```python
from build123d import *

# Parameters (mm, degrees)
SKETCH1_R           = 2.54
BOSS_EXTRUDE1_DEPTH = 0.8128
SKETCH2_R           = 2.54
CUT_EXTRUDE1_DEPTH  = 118.606454516
SKETCH3_R           = 2.54
CUT_EXTRUDE2_DEPTH  = 118.606454516


with BuildPart() as part:
    # Sketch1 → Boss-Extrude1 (new body)
    with BuildSketch(Plane(origin=(0, 0, 0), x_dir=(1, 0, 0), z_dir=(0, 1, 0))):
        Polygon((0, 88.9), (-76.989658396, 44.45), (-76.989658396, -44.45), (0, -88.9), (76.989658396, -44.45), (76.989658396, 44.45), align=None)
        with Locations(Location((13.322783942, -73.875738686, 0), (0, 0, 270))):
            Circle(SKETCH1_R, mode=Mode.SUBTRACT)
        with Locations(Location((24.32130657, -67.525738686, 0), (0, 0, 270))):
            Circle(SKETCH1_R, mode=Mode.SUBTRACT)
        with Locations(Location((-70.639658396, 12.7, 0), (0, 0, 270))):
            Circle(SKETCH1_R, mode=Mode.SUBTRACT)
        with Locations(Location((-70.639658396, 25.4, 0), (0, 0, 270))):
            Circle(SKETCH1_R, mode=Mode.SUBTRACT)
        with Locations(Location((46.318351826, 54.825738686, 0), (0, 0, 270))):
            Circle(SKETCH1_R, mode=Mode.SUBTRACT)
        with Locations(Location((57.316874454, 48.475738686, 0), (0, 0, 270))):
            Circle(SKETCH1_R, mode=Mode.SUBTRACT)
    extrude(amount=BOSS_EXTRUDE1_DEPTH)

    # Sketch2 → Cut-Extrude1 (cut, through all)
    with BuildSketch(Plane(origin=(0, 0.8128, 0), x_dir=(1, 0, 0), z_dir=(0, 1, 0))):
        with Locations(Location((28.620590949, 59.732317666, 0), (0, 0, 270))):
            Circle(SKETCH2_R)
        with Locations(Location((48.416295038, -22.82051708, 0), (0, 0, 270))):
            Circle(SKETCH2_R)
        with Locations(Location((-52.77011314, 35.59948292, 0), (0, 0, 270))):
            Circle(SKETCH2_R)
        with Locations(Location((-32.974409051, -46.953351826, 0), (0, 0, 270))):
            Circle(SKETCH2_R)
    extrude(amount=-CUT_EXTRUDE1_DEPTH, mode=Mode.SUBTRACT)

    # Sketch3 → Cut-Extrude2 (cut, through all)
    with BuildSketch(Plane(origin=(0, 0.8128, 0), x_dir=(1, 0, 0), z_dir=(0, 1, 0))):
        with Locations(Location((-7.823522628, -77.050738686, 0), (0, 0, 270))):
            Circle(SKETCH3_R)
        with Locations(Location((-62.816135768, -45.300738686, 0), (0, 0, 270))):
            Circle(SKETCH3_R)
        with Locations(Location((-56.466135768, -34.302216058, 0), (0, 0, 270))):
            Circle(SKETCH3_R)
        with Locations(Location((-1.473522628, -66.052216058, 0), (0, 0, 270))):
            Circle(SKETCH3_R)
    extrude(amount=-CUT_EXTRUDE2_DEPTH, mode=Mode.SUBTRACT)


solid = part.part
```
CAD build for the part. Positions are in the model's coordinates, mm. Round coordinates to 2 decimals unless told otherwise and drop trailing zeros. Write each loop counter-clockwise with the first axis right and the second up, starting at its lowest first coordinate (ties: lowest second). Pieces come first, ordered by that corner, then holes. Notation, with made-up numbers: (-9, -31) - (2, -31) arc R26 ccw to (2, -3) - close; hole circle Ø6 at (64, 36.5). An arc over 180 degrees is marked (long way). Write item = value, one per line. Start each with the question number.
Q1. Band-saw the part on D-D (z = -74.5). Give the cut face in (x, y).
Q2. Drop a flat-ended pin along its axis: pin 1 (4.5 mm diameter, centred on x = -70.64, z = -25.4, fed in from -Y). Give the stop position or say it passes through.
Q3. Mould opens along Z. For faces 1 (the cylindrical face through (-60.674, 0.412, 46.666)), 2 (the flat face through (37.956, 0.401, 66.986)), 3 (the flat face through (-1, 0, -1)) say: pulls with the +Z half, pulls with the -Z half, needs draft (parallel to the pull), parting line crosses it, or undercut.
Q4. Probe L1, parallel to Z at x = -55, y = 0.45; L2, parallel to Z at x = 58.5, y = 0.15 (3 decimals); L3, parallel to Z at x = -32, y = 0.65. List the from-to ranges inside material, lowest first. Write a range as from..to.
Q5. Band-saw the part on A-A (z = -12.7). Give the cut face in (x, y), then the cut area to 3 significant figures.
Q6. Band-saw the part on C-C (x = -24). Give the cut face in (y, z).
Q7. Band-saw the part on B-B (y = 0.2). Count the separate pieces of the cut face and the enclosed holes in it, then the cut area to 3 significant figures.
Answers below:
q1.outline = (-24.94, 0) - (24.94, 0) - (24.94, 0.81) - (-24.94, 0.81) - close
q2.pin_1 = through
q3.face_1 = undercut
q3.face_2 = pulls with the +Z half
q3.face_3 = needs draft
q4.L1 = -57.15..-36.82, -34.38..32.23, 36.38..57.15
q4.L2 = -55.125..-50.723, -46.228..55.125
q4.L3 = -70.42..44.61, 49.3..70.42
q5.outline = (-76.99, 0) - (-73.18, 0) - (-73.18, 0.81) - (-76.99, 0.81) - close; (-68.1, 0) - (76.99, 0) - (76.99, 0.81) - (-68.1, 0.81) - close
q5.area = 121 mm2
q6.outline = (0, -75.04) - (0.81, -75.04) - (0.81, 75.04) - (0, 75.04) - close
q7.separate_pieces = 1
q7.enclosed_holes = 14
q7.area = 20,200 mm2
